```python
from build123d import *

# Parameters (mm, degrees)
F0_R     = 1.6
F1_DEPTH = 2
F3_DEPTH = 1
F4_R     = 0.5


with BuildPart() as f1:
    # F0 (on Front) → F1 (new body)
    with BuildSketch(Plane.XZ):
        with BuildLine():
            Line((2.5, 44), (0, 44))
            Line((0, 44), (-2.5, 44))
            ThreePointArc((-2.5, 44), (-5.6819805153, 42.6819805153), (-7, 39.5))
            Line((-7, 39.5), (-7, 19.5))
            ThreePointArc((-7, 19.5), (-8.6109127035, 15.6109127035), (-12.5, 14))
            Line((-12.5, 14), (-17.5, 14))
            ThreePointArc((-17.5, 14), (-20.6819805153, 12.6819805153), (-22, 9.5))
            Line((-22, 9.5), (-22, 4.5))
            ThreePointArc((-22, 4.5), (-20.6819805153, 1.3180194847), (-17.5, 0))
            Line((-17.5, 0), (0, 0))
            Line((0, 0), (17.5, 0))
            ThreePointArc((17.5, 0), (20.6819805153, 1.3180194847), (22, 4.5))
            Line((22, 4.5), (22, 9.5))
            ThreePointArc((22, 9.5), (20.6819805153, 12.6819805153), (17.5, 14))
            Line((17.5, 14), (12.5, 14))
            ThreePointArc((12.5, 14), (8.6109127035, 15.6109127035), (7, 19.5))
            Line((7, 19.5), (7, 39.5))
            ThreePointArc((7, 39.5), (5.6819805153, 42.6819805153), (2.5, 44))
        make_face()
        with Locations((-15, 7)):
            Circle(F0_R, mode=Mode.SUBTRACT)
        with Locations((0, 7)):
            Circle(F0_R, mode=Mode.SUBTRACT)
        with Locations((15, 7)):
            Circle(F0_R, mode=Mode.SUBTRACT)
        with Locations((0, 22)):
            Circle(F0_R, mode=Mode.SUBTRACT)
        with Locations((0, 37)):
            Circle(F0_R, mode=Mode.SUBTRACT)
    extrude(amount=F1_DEPTH)

    # F2 (on face) → F3 (join)
    with BuildSketch(Plane.XZ.offset(2)):
        with BuildLine():
            ThreePointArc((22, 9.5), (20.6819805153, 12.6819805153), (17.5, 14))
            Line((17.5, 14), (12.5, 14))
            ThreePointArc((12.5, 14), (8.6109127035, 15.6109127035), (7, 19.5))
            Line((7, 19.5), (7, 39.5))
            ThreePointArc((7, 39.5), (5.6819805153, 42.6819805153), (2.5, 44))
            Line((2.5, 44), (-2.5, 44))
            ThreePointArc((-2.5, 44), (-5.6819805153, 42.6819805153), (-7, 39.5))
            Line((-7, 39.5), (-7, 19.5))
            ThreePointArc((-7, 19.5), (-8.6109127035, 15.6109127035), (-12.5, 14))
            Line((-12.5, 14), (-17.5, 14))
            ThreePointArc((-17.5, 14), (-20.6819805153, 12.6819805153), (-22, 9.5))
            Line((-22, 9.5), (-22, 4.5))
            ThreePointArc((-22, 4.5), (-20.6819805153, 1.3180194847), (-17.5, 0))
            Line((-17.5, 0), (17.5, 0))
            ThreePointArc((17.5, 0), (20.6819805153, 1.3180194847), (22, 4.5))
            Line((22, 4.5), (22, 9.5))
        make_face()
        with BuildLine():
            Line((-5.5, 19.5), (-5.5, 39.5))
            ThreePointArc((-5.5, 39.5), (-4.6213203436, 41.6213203436), (-2.5, 42.5))
            Line((-2.5, 42.5), (2.5, 42.5))
            ThreePointArc((2.5, 42.5), (4.6213203436, 41.6213203436), (5.5, 39.5))
            Line((5.5, 39.5), (5.5, 19.5))
            ThreePointArc((5.5, 19.5), (7.5502525317, 14.5502525317), (12.5, 12.5))
            Line((12.5, 12.5), (17.5, 12.5))
            ThreePointArc((17.5, 12.5), (19.6213203436, 11.6213203436), (20.5, 9.5))
            Line((20.5, 9.5), (20.5, 4.5))
            ThreePointArc((20.5, 4.5), (19.6213203436, 2.3786796564), (17.5, 1.5))
            Line((17.5, 1.5), (-17.5, 1.5))
            ThreePointArc((-17.5, 1.5), (-19.6213203436, 2.3786796564), (-20.5, 4.5))
            Line((-20.5, 4.5), (-20.5, 9.5))
            ThreePointArc((-20.5, 9.5), (-19.6213203436, 11.6213203436), (-17.5, 12.5))
            Line((-17.5, 12.5), (-12.5, 12.5))
            ThreePointArc((-12.5, 12.5), (-7.5502525317, 14.5502525317), (-5.5, 19.5))
        make_face(mode=Mode.SUBTRACT)
    extrude(amount=F3_DEPTH)

    # F4
    f4_edges = [f1.edges().sort_by_distance(p)[0] for p in [
        (-7, -3, 29.5),
        (-5.5, -3, 29.5),
    ]]
    fillet(f4_edges, radius=F4_R)


solid = f1.part
```
Model file for the job. Use its own axes, mm. A direction names the side the tool comes from. Give positions to 0.01 mm unless a question says otherwise; leave off trailing zeros. Loops run counter-clockwise (first coordinate to the right, second up) from the corner with the lowest first, then second, coordinate; pieces in that order, holes last. Notation, with made-up numbers: M 54.5,72 L 81.5,72 A26 ccw 81.5,93 Z; hole C 59,-24.75 d3. An arc over 180 degrees is marked long. Use one line per item in the form item = value.
Item 1: Slice it at D-D on z = 22. List the corners of the cut face in (x, y).
Filled in:
outline = M -7,-2.5 A0.5 ccw -6.5,-3 L -6,-3 A0.5 ccw -5.5,-2.5 L -5.5,-2 L -1.6,-2 L -1.6,0 L -7,0 Z; M 1.6,-2 L 5.5,-2 L 5.5,-2.5 A0.5 ccw 6,-3 L 6.5,-3 A0.5 ccw 7,-2.5 L 7,0 L 1.6,0 Z
Item 2: Slice it at B-B on x = 15. List the corners of the cut face in (y, z), and give its area (3 significant figures).
Filled in:
outline = M -3,0.5 A0.5 ccw -2.5,0 L 0,0 L 0,5.4 L -2,5.4 L -2,1.5 L -2.5,1.5 A0.5 ccw -3,1 Z; M -3,13 A0.5 ccw -2.5,12.5 L -2,12.5 L -2,8.6 L 0,8.6 L 0,14 L -2.5,14 A0.5 ccw -3,13.5 Z
area = 24.4 mm^2
Item 3: Slice it at C-C on x = 0. List the corners of the cut face in (y, z).
Filled in:
outline = M -3,0.5 A0.5 ccw -2.5,0 L 0,0 L 0,5.4 L -2,5.4 L -2,1.5 L -2.5,1.5 A0.5 ccw -3,1 Z; M -3,43 A0.5 ccw -2.5,42.5 L -2,42.5 L -2,38.6 L 0,38.6 L 0,44 L -2.5,44 A0.5 ccw -3,43.5 Z; M -2,8.6 L 0,8.6 L 0,20.4 L -2,20.4 Z; M -2,23.6 L 0,23.6 L 0,35.4 L -2,35.4 Z
Item 4: Which spindle directions (+Z, -Z, +X, -X, +Y, -Y) get a long thin tool onto all of the face, cutting with end or side? Do faces 1 (the cylindrical face through (4.6, -2.25, 41.64)), 2 (the cylindrical face through (0.74, -0.99, 35.58)), 3 (the flat face through (-15, -1, 14)). Say none if no direction does.
Filled in:
face_1 = -Y
face_2 = +Y, -Y
face_3 = +Z, -X, +Y, -Y
Item 5: Slice it at A-A on z = 7. List the corners of the cut face in (x, y).
Filled in:
outline = M -22,-2.5 A0.5 ccw -21.5,-3 L -21,-3 A0.5 ccw -20.5,-2.5 L -20.5,-2 L -16.6,-2 L -16.6,0 L -22,0 Z; M -13.4,-2 L -1.6,-2 L -1.6,0 L -13.4,0 Z; M 1.6,-2 L 13.4,-2 L 13.4,0 L 1.6,0 Z; M 16.6,-2 L 20.5,-2 L 20.5,-2.5 A0.5 ccw 21,-3 L 21.5,-3 A0.5 ccw 22,-2.5 L 22,0 L 16.6,0 Z
Item 6: Two-plate mould, pull along Z, no slides. Class faces 4 (the flat face through (7, -1, 29)), 5 (the cylindrical face through (20.647, -1.232, 1.283)), 6 (the flat face through (0, -2, 18)): released by +Z, released by -Z, zero draft, split by the parting line, or undercut.
Filled in:
face_4 = zero draft
face_5 = released by -Z
face_6 = undercut
Item 7: Drill centre lines: L1, parallel to Z at x = 0, y = -1.45; L2, parallel to X at y = -2.4, z = 30.5; L3, parallel to Z at x = -16.5, y = -2.2. Where is each one in solid material? Low to high.
Filled in:
L1 = 0 to 5.4, 8.6 to 20.4, 23.6 to 35.4, 38.6 to 44
L2 = -7 to -5.5, 5.5 to 7
L3 = 0 to 1.5, 12.5 to 14
Item 8: Flat gauge pins, fed straight in: pin 1 Ø0.6 at (x, y) = (6, -2.5) entering from +Z; pin 2 Ø1 at (y, z) = (-2, 30.5) entering from +X; pin 3 Ø1.2 at (x, y) = (-14.5, -1) entering from +Z; pin 4 Ø8 at (x, z) = (4.5, 18) entering from +Y. Where does each tip first touch, or does it go through?
Filled in:
pin_1 = 42.66
pin_2 = 7
pin_3 = 14
pin_4 = 0
